Part model, mm, in its own coordinate system. Give positions to 0.01 mm unless a question says otherwise; leave off trailing zeros. Order: outer loops, then holes, each group sorted by start corner. A loop starts at its lowest first (then second) coordinate and runs counter-clockwise, first axis right, second up. Notation, with made-up numbers: (6, 53.25) - (37, 53.25) arc R28 ccw to (37, 77.25) - close; hole circle Ø2 at (-27, 8). An arc over 180 degrees is marked (long way). One line per item, written item: value.
```python
from build123d import *

# Parameters (mm, degrees)
SKETCH_1_R      = 1.25
SKETCH_1_R_2    = 15.5
EXTRUDE_1_DEPTH = 16
FILLET_1_R      = 4


with BuildPart() as part:
    # Эскиз1 → Бобышка-Вытянуть1 (new body)
    with BuildSketch(Plane(origin=(0, 0, 0), x_dir=(1, 0, 0), z_dir=(0, 1, 0))):
        with BuildLine():
            Line((-14.641038215, -21), (14.641038215, -21))
            ThreePointArc((14.641038215, -21), (18.101933598, -18.101933598), (21, -14.641038215))
            Line((21, -14.641038215), (21, 14.641038215))
            ThreePointArc((21, 14.641038215), (18.101933598, 18.101933598), (14.641038215, 21))
            Line((14.641038215, 21), (-14.641038215, 21))
            ThreePointArc((-14.641038215, 21), (-18.101933598, 18.101933598), (-21, 14.641038215))
            Line((-21, 14.641038215), (-21, -14.641038215))
            ThreePointArc((-21, -14.641038215), (-18.101933598, -18.101933598), (-14.641038215, -21))
        make_face()
        with Locations((-15.5, 15.5)):
            Circle(SKETCH_1_R, mode=Mode.SUBTRACT)
        with Locations((15.5, 15.5)):
            Circle(SKETCH_1_R, mode=Mode.SUBTRACT)
        with Locations((15.5, -15.5)):
            Circle(SKETCH_1_R, mode=Mode.SUBTRACT)
        with Locations((-15.5, -15.5)):
            Circle(SKETCH_1_R, mode=Mode.SUBTRACT)
        Circle(SKETCH_1_R_2, mode=Mode.SUBTRACT)
    extrude(amount=EXTRUDE_1_DEPTH)

    # Скругление1
    fillet_1_edges = [part.edges().sort_by_distance(p)[0] for p in [
        (21, 8, -14.641038215),
        (21, 8, 14.641038215),
        (14.641038215, 8, 21),
        (-14.641038215, 8, 21),
        (-21, 8, 14.641038215),
        (-21, 8, -14.641038215),
        (-14.641038215, 8, -21),
        (14.641038215, 8, -21),
    ]]
    fillet(fillet_1_edges, radius=FILLET_1_R)


solid = part.part
```
1) Cut at C-C, the plane x = -9. Give the cut face in (y, z), then the cut area to 3 significant figures.
Outcome:
outline: (0, -21) - (16, -21) - (16, -12.62) - (0, -12.62) - close; (0, 12.62) - (16, 12.62) - (16, 21) - (0, 21) - close
area: 268 mm^2
2) Drill centre lines: line 1 along Z through (x, y) = (0, 10.75); line 2 along X through (y, z) = (11.75, 11.5). Where is each one in solid material? Low to high. Write a range as from..to.
Outcome:
line 1: z = -21..-15.5, 15.5..21
line 2: x = -21..-10.39, 10.39..21
3) Cut at A-A, the plane z = 0. Give the cut face in (x, y), then the cut area to 3 significant figures.
Outcome:
outline: (-21, 0) - (-15.5, 0) - (-15.5, 16) - (-21, 16) - close; (15.5, 0) - (21, 0) - (21, 16) - (15.5, 16) - close
area: 176 mm^2
4) Mould opens along X. For faces 1 (the cylindrical face through (-2.018, 7.888, -15.368)), 2 (the flat face through (9, 0, 14)), 3 (the cylindrical face through (20.775, 8.112, 14.648)), 4 (the cylindrical face through (-18.071, 7.888, -18.132)) say: released by +X, released by -X, zero draft, split by the parting line, or undercut.
Outcome:
face 1: undercut
face 2: zero draft
face 3: released by +X
face 4: released by -X
5) Cut at B-B, the plane y = 9. Give the cut face in (x, z).
Outcome:
outline: (-21, -13.33) arc R4 ccw to (-20.15, -15.79) arc R25.6 ccw to (-15.79, -20.15) arc R4 ccw to (-13.33, -21) - (13.33, -21) arc R4 ccw to (15.79, -20.15) arc R25.6 ccw to (20.15, -15.79) arc R4 ccw to (21, -13.33) - (21, 13.33) arc R4 ccw to (20.15, 15.79) arc R25.6 ccw to (15.79, 20.15) arc R4 ccw to (13.33, 21) - (-13.33, 21) arc R4 ccw to (-15.79, 20.15) arc R25.6 ccw to (-20.15, 15.79) arc R4 ccw to (-21, 13.33) - close; hole circle Ø2.5 at (-15.5, -15.5); hole circle Ø2.5 at (-15.5, 15.5); hole circle Ø31 at (0, 0); hole circle Ø2.5 at (15.5, -15.5); hole circle Ø2.5 at (15.5, 15.5)
6) Cut at D-D, the plane z = -15. Give the cut face in (x, y).
Outcome:
outline: (-20.63, 0) - (-16.65, 0) - (-16.65, 16) - (-20.63, 16) - close; (-14.35, 0) - (-3.91, 0) - (-3.91, 16) - (-14.35, 16) - close; (3.91, 0) - (14.35, 0) - (14.35, 16) - (3.91, 16) - close; (16.65, 0) - (20.63, 0) - (20.63, 16) - (16.65, 16) - close
